from build123d import *

# Parameters (mm, degrees)
F0_W     = 44
F0_H     = 34
F0_W_2   = 30
F0_H_2   = 22.5
F1_DEPTH = 2
F3_W     = 44
F3_H     = 3
F6_DEPTH = 2.5
F9_W     = 3
F9_H     = 5


with BuildPart() as f1:
    # F0 (on Right) → F1 (new body)
    with BuildSketch(Plane.YZ):
        Rectangle(F0_W, F0_H)
        with Locations((0, 0.75)):
            Rectangle(F0_W_2, F0_H_2, mode=Mode.SUBTRACT)
    extrude(amount=F1_DEPTH)

    # F4: sweep along a path in F2
    with BuildLine(Plane.XZ.offset(22)) as f4_path:
        ThreePointArc((0, -17), (-13.5188817396, -16.4097528762), (-24.931453195, -23.6803627497))
    # F3 (on face) → F4 (sweep)
    with BuildSketch(Plane(origin=(0, 0, 0), x_dir=(0, -1, 0), z_dir=(-1, 0, 0))):
        with Locations((0, -15.5)):
            Rectangle(F3_W, F3_H)
    sweep(path=f4_path.line)

    # F5 (on face) → F6 (join)
    with BuildSketch(Plane.XZ.offset(22)):
        with BuildLine():
            Line((0, -14), (0, 17))
            Line((0, 17), (-27.7505310574, -22.6543023198))
            ThreePointArc((-27.7505310574, -22.6543023198), (-15.2396110487, -13.9522967433), (0, -14))
        make_face()
    extrude(amount=-F6_DEPTH)


with BuildPart() as f7_1:
    # F7: instance of F1
    add(f1.part.mirror(Plane.XZ))


with BuildPart() as f1_1:
    add(f1.part)

    # F8: union F7_1
    add(f7_1.part)

    # F10: sweep along a path in F2
    with BuildLine(Plane.XZ.offset(22)) as f10_path:
        ThreePointArc((-24.931453195, -23.6803627497), (-10.8151434968, -15.8604105956), (4.9059770967, -19.5029671802))
    # F9 (on face) → F10 (sweep, cut)
    with BuildSketch(Plane(origin=(-10.5271478923, 0, -28.9231011252), x_dir=(0.9396926208, 0, -0.3420201433), z_dir=(-0.3420201433, 0, -0.9396926208))):
        with Locations((-18.8287415311, -14.5)):
            Rectangle(F9_W, F9_H)
        with Locations((-18.8287415311, 14.5)):
            Rectangle(F9_W, F9_H)
    sweep(path=f10_path.line, mode=Mode.SUBTRACT)


solid = f1_1.part
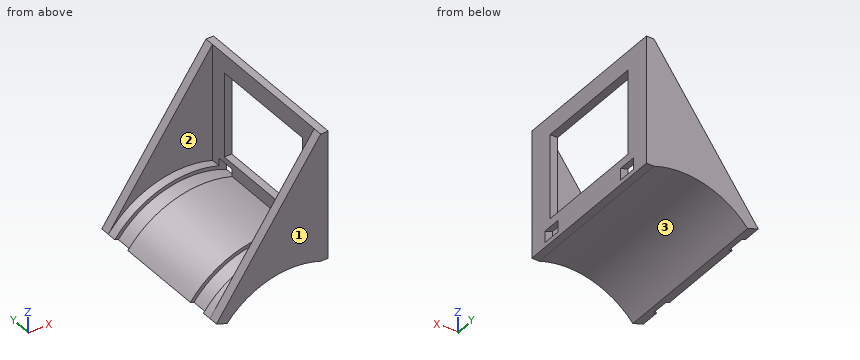
CAD build for the part. Positions are in the model's coordinates, mm. Face numbers are marked on the shaded views. Give positions to 0.01 mm unless a question says otherwise; leave off trailing zeros. Loops run counter-clockwise (first coordinate to the right, second up) from the corner with the lowest first, then second, coordinate; pieces in that order, holes last. Notation, with made-up numbers: M 70.5,72.5 L 115.5,72.5 A21 ccw 115.5,106.5 Z; hole C 76,15.5 d2. An arc over 180 degrees is marked long. One line per question, with ' | ' between items. Start each with the question number.
1. Saw through at B-B on z = 5. Give the cut face in (x, y).
2. Probe L1, parallel to Y at x = -1.5, z = -2; L2, parallel to Y at x = 0.5, z = 10.5; L3, parallel to X at y = 8.5, z = -11. List the from-to ranges inside material, lowest first. Write a range as from..to.
3. Two-plate mould, pull along Y, no slides. Class the marked faces 1, 2 and 3: pulls with the +Y half, pulls with the -Y half, needs draft (parallel to the pull), parting line crosses it, or undercut.
4. Saw through at C-C on y = -13. Give the cut face in (x, z).
5. Saw through at D-D on x = -18. Give the cut face in (y, z), plus the area to 3 significant figures.
6. Flat gauge pins, fed straight in: pin 1 (0.6 mm diameter, centred on x = 0.5, y = -7.5, fed in from -Z); pin 2 (1.5 mm diameter, centred on x = -17.5, y = 10.5, fed in from +Z); pin 3 (15.5 mm diameter, centred on y = -3.5, z = 2.5, fed in from -X); pin 4 (3 mm diameter, centred on x = -4, y = 16.5, fed in from +Z). Where does each tip first touch, or does it go through?
7. Saw through at A-A on y = -4. Give the cut face in (x, z), plus the area to 3 significant figures.
Result sheet:
1) outline: M -8.4,-22 L 2,-22 L 2,-15 L 0,-15 L 0,-19.5 L -8.4,-19.5 Z; M -8.4,19.5 L 0,19.5 L 0,15 L 2,15 L 2,22 L -8.4,22 Z
2) L1: y = -22..-19.5, 19.5..22 | L2: y = -22..-15, 15..22 | L3: x = 0..2
3) face 1: pulls with the -Y half | face 2: undercut | face 3: needs draft
4) outline: M -26.81,-23 L -24.93,-23.68 A22.5 cw 0,-17 L 2,-17 L 2,-15.76 A24.39 ccw Z; M 0,-12 A27.25 cw 2,-12.67 L 2,-10.5 L 0,-10.5 Z; M 0,12 L 2,12 L 2,17 L 0,17 Z
5) outline: M -22,-18.14 L 22,-18.14 L 22,-8.72 L 19.5,-8.72 L 19.5,-14.99 L 17,-14.99 L 17,-16.04 L 12,-16.04 L 12,-14.99 L -12,-14.99 L -12,-16.04 L -17,-16.04 L -17,-14.99 L -19.5,-14.99 L -19.5,-8.72 L -22,-8.72 Z | area: 159 mm^2
6) pin 1: stops at z = -17 | pin 2: stops at z = -14.48 | pin 3: passes through | pin 4: stops at z = -12.91
7) outline: M -27.75,-22.65 L -24.93,-23.68 A22.5 cw 0,-17 L 2,-17 L 2,-10.5 L 0,-10.5 L 0,-14 A25.34 ccw Z; M 0,12 L 2,12 L 2,17 L 0,17 Z | area: 106 mm^2
